Could you check a few things on this model? Use its own coordinates, in mm. Face numbers are marked on the shaded views. A direction names the side the tool comes from. Coordinates: 2 decimals unless noted, no trailing zeros. Loops run counter-clockwise (first coordinate to the right, second up) from the corner with the lowest first, then second, coordinate; pieces in that order, holes last. Notation, with made-up numbers: (59, 63) - (79, 63) arc R20 cw to (79, 93) - close; hole circle Ø5 at (44, 53.25). An arc over 180 degrees is marked (long way). One line per item, written item: value. Start each with the question number.
(1) On a 3-axis mill with a long thin cutter (end or side, diameter ignored), from which of +Z, -Z, +X, -X, +Y, -Y can I reach the whole of each face in a straight line? I mean the marked faces 1, 2 and 3. Say none if no direction works.
(2) If we section it at C-C on z = -1.8: Write out the boundary of the cut face in (x, y).
(3) If we section it at D-D on z = 1.5: Write out the boundary of the cut face in (x, y).
(4) If I drill on line 1 along Z through (x, y) = (-1.75, 3.7); line 2 along X through (y, z) = (3, 0); line 3 along Z through (x, y) = (2, 3.75), over which ranges is the centre line in solid material (lowest first)? Write a range as from..to.
(5) If we mould it in two halves opening along X, with no side actions, what happens to the marked faces 4, 5 and 6? For each: pulls with the +X half, pulls with the -X half, needs draft (parallel to the pull), parting line crosses it, or undercut.
(6) If we section it at A-A on x = 2.25: Write out the boundary of the cut face in (y, z), then the cut area to 3 significant figures.
(7) If we section it at B-B on y = 0.6: Write out the boundary of the cut face in (x, z), then the cut area to 3 significant figures.
(8) I'm going to push flat-ended pins straight in: P1, Ø1.5, axis at x = -0.5, z = 1, coming from the +Y side; P2, Ø2.5, axis at x = 2, y = 3, coming from the +Z side; P3, Ø0.9, axis at x = -2, y = 2.5, coming from the +Z side. Where does each tip first touch, or does it pass through?
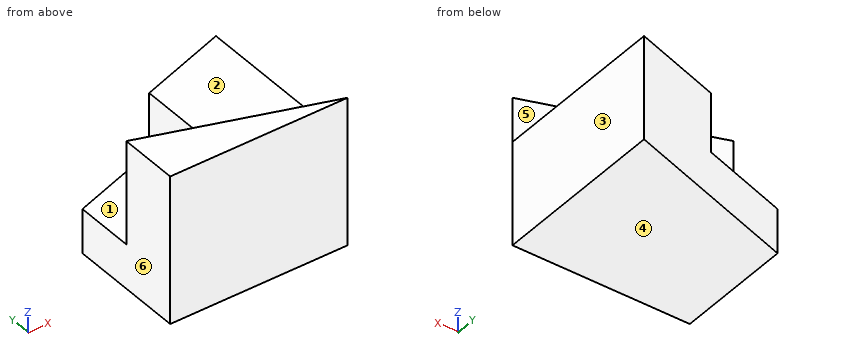
```python
from build123d import *

# Parameters (mm, degrees)
SKETCH1_W           = 6
SKETCH1_H           = 5
BOSS_EXTRUDE1_DEPTH = 6
CUT_EXTRUDE1_DEPTH  = 3.5
CUT_EXTRUDE2_DEPTH  = 1.5
CUT_EXTRUDE3_DEPTH  = 11.5


with BuildPart() as part:
    # Sketch1 → Boss-Extrude1 (new body)
    with BuildSketch(Plane(origin=(0, 0, 0), x_dir=(1, 0, 0), z_dir=(0, 1, 0))):
        Rectangle(SKETCH1_W, SKETCH1_H)
    extrude(amount=BOSS_EXTRUDE1_DEPTH)

    # Sketch2 → Cut-Extrude1 (cut)
    with BuildSketch(Plane.XY.offset(2.5)):
        Polygon((-3, 6), (-3, 2), (0, 1), (0, 6), align=None)
    extrude(amount=-CUT_EXTRUDE1_DEPTH, mode=Mode.SUBTRACT)

    # Sketch3 → Cut-Extrude2 (cut)
    with BuildSketch(Plane.XY.offset(2.5)):
        Polygon((0, 1), (3, 0), (3, 6), (0, 6), align=None)
    extrude(amount=-CUT_EXTRUDE2_DEPTH, mode=Mode.SUBTRACT)

    # Sketch4 → Cut-Extrude3 (cut)
    with BuildSketch(Plane.XY.offset(1)):
        Polygon((3, 6), (-3, 4), (-3, 6), align=None)
    extrude(amount=-CUT_EXTRUDE3_DEPTH, mode=Mode.SUBTRACT)


solid = part.part
```
Values:
1. face 1: +Z, +Y
1. face 2: +Z, +X, +Y
1. face 3: +Z, -Z, +X, +Y, -Y
2. outline: (-3, 0) - (3, 0) - (3, 6) - (-3, 4) - close
3. outline: (-3, 0) - (3, 0) - (-3, 2) - close
4. line 1: z = -2.5..-1
4. line 2: x = 0..3
4. line 3: z = -2.5..1
5. face 4: needs draft
5. face 5: undercut
5. face 6: pulls with the -X half
6. outline: (0, -2.5) - (5.75, -2.5) - (5.75, 1) - (0.25, 1) - (0.25, 2.5) - (0, 2.5) - close
6. area: 20.5 mm2
7. outline: (-3, -2.5) - (3, -2.5) - (3, 1) - (1.2, 1) - (1.2, 2.5) - (-3, 2.5) - close
7. area: 27.3 mm2
8. P1: stops at y = 5.08
8. P2: stops at z = 1
8. P3: stops at z = -1
